Verification items for the finished model (mm, model axes). Face numbers are marked on the shaded views. A direction names the side the tool comes from. Give positions to 0.01 mm unless a question says otherwise; leave off trailing zeros. Loops run counter-clockwise (first coordinate to the right, second up) from the corner with the lowest first, then second, coordinate; pieces in that order, holes last. Notation, with made-up numbers: M 42,51 L 57,51 A17 ccw 57,78 Z; hole C 73.5,16 d3. An arc over 180 degrees is marked long. Use a Markdown table: item, result.
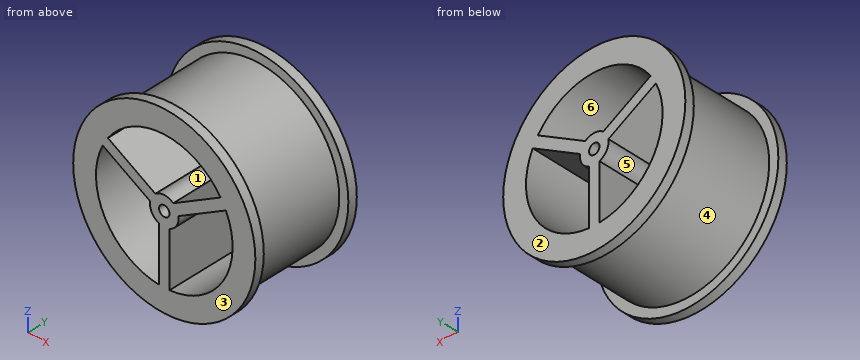
Autodesk Inventor part; units mm, degrees
ref_plane "YZ Plane" through (0, 0, 0) normal (1, 0, 0) x (0, 1, 0)
ref_plane "XZ Plane" through (0, 0, 0) normal (0, 1, 0) x (-1, 0, 0)
ref_plane "XY Plane" through (0, 0, 0) normal (0, 0, 1) x (1, 0, 0)
sketch "Эскиз1" plane through (0, 0, 0) normal (0, 0, 1) x (1, 0, 0)
  line L0 (0, 0) -> (15, 0)
  line L1 (15, 0) -> (15, 10)
  line L2 (15, 10) -> (15, -10)
  line L3 (15, 10) -> (18, 10)
  line L4 (18, 10) -> (18, -10)
  line L5 (18, -10) -> (15, -10)
  line L6 (15, -10) -> (15, 10)
  line L7 (15, 10) -> (20, 10)
  line L8 (20, 10) -> (20, 12)
  line L9 (20, 12) -> (15, 12)
  line L10 (15, 12) -> (15, 10)
  line L11 (15, -10) -> (20, -10)
  line L12 (20, -10) -> (20, -12)
  line L13 (20, -12) -> (15, -12)
  line L14 (15, -12) -> (15, -10)
  line L15 (0, 0) -> (0, 10)
  dimension "d0" = 15
  dimension "d1" = 10
  dimension "d2" = 20
  dimension "d3" = 3
  dimension "d4" = 5
  dimension "d5" = 2
  dimension "d6" = 5
  dimension "d7" = 2
revolve "Вращение1" add sketch "Эскиз1" angle 360 about axis through (0, 0, 0) along (0, 1, 0)
sketch "Эскиз2" plane through (0, -12, 0) normal (0, -1, 0) x (1, 0, 0)
  circle A0 centre (0, 0) radius 1.15
  circle A1 centre (0, 0) radius 3.15
  circle A2 centre (0, 0) radius 15
  line L0 (-1.15, 0) -> (1.15, 0)
  line L1 (1.15, 0) -> (1.15, -15.6419)
  line L2 (1.15, -15.6419) -> (-1.15, -15.6419)
  line L3 (-1.15, -15.6419) -> (-1.15, 0)
  line L4 (14.1213, 6.825) -> (0.575, -0.9959)
  line L5 (-0.575, 0.9959) -> (12.9713, 8.8169)
  line L6 (12.9713, 8.8169) -> (14.1213, 6.825)
  line L7 (0.575, -0.9959) -> (-0.575, 0.9959)
  line L8 (-12.9713, 8.8169) -> (0.575, 0.9959)
  line L9 (-0.575, -0.9959) -> (-14.1213, 6.825)
  line L10 (-14.1213, 6.825) -> (-12.9713, 8.8169)
  line L11 (0.575, 0.9959) -> (-0.575, -0.9959)
  dimension "d9" = 2.3
  dimension "d10" = 2
  dimension "d13" = 360
extrude "Выдавливание1" add sketch "Эскиз2" against normal up to surface (24 mm away) contours L0 L11 A0 | L1 L4 A0 | A0 L7 L0 | A0 L8 L5 A1 L4 L1 | L11 L7 A0 | A0 L5 L8 | L4 L1 A1 L3 L9 A0 | A0 L11 L7 | L11 A0 L0 | L0 A0 L7 | L4 A1 L1 | A0 L3 L9 A1 L8 L5 | L8 A1 L5 | L9 L3 A0 | L1 A2 L3 A1 | A1 L5 A2 L4 | A1 L9 A2 L8 | L3 A1 L9 | L1 L2 L3 A2 | A2 L5 L6 L4 | A2 L9 L10 L8
extrude "Выдавливание2" cut sketch "Эскиз2" against normal up to surface (24 mm away) contours L0 L11 A0 | A0 L7 L0 | L11 L7 A0 | A0 L11 L7 | L11 A0 L0 | L0 A0 L7
properties part number "Wheel down"
(1) Gauge pin test, flat ends, axial feed: P1, Ø12, axis at x = -3.5, y = 9, coming from the -Z side; P2, Ø2, axis at x = -10.5, y = 8, coming from the +Z side; P3, Ø1.5, axis at x = 3, y = -3.5, coming from the -Z side. Record the tip position at first contact, or that the pin passes through.
Results below:
| item | result |
|---|---|
| P1 | z = -20 |
| P2 | z = 15.29 |
| P3 | z = -17.86 |
(2) Cross-section at D-D on z = 9.5. Record the cut outline in (x, y), then the cut area to 3 significant figures.
Results below:
| item | result |
|---|---|
| outline | M -17.6,-12 L -11.61,-12 L -11.61,12 L -17.6,12 L -17.6,10 L -15.29,10 L -15.29,-10 L -17.6,-10 Z; M 11.61,-12 L 17.6,-12 L 17.6,-10 L 15.29,-10 L 15.29,10 L 17.6,10 L 17.6,12 L 11.61,12 Z |
| area | 195 mm^2 |
(3) Cross-section at A-A on x = 0. Record the cut outline in (y, z), then the cut area to 3 significant figures.
Results below:
| item | result |
|---|---|
| outline | M -12,-20 L -10,-20 L -10,-18 L 10,-18 L 10,-20 L 12,-20 L 12,-1.15 L -12,-1.15 Z; M -12,1.15 L 12,1.15 L 12,3.15 L -12,3.15 Z; M -12,15 L 12,15 L 12,20 L 10,20 L 10,18 L -10,18 L -10,20 L -12,20 Z |
| area | 540 mm^2 |
(4) Draft check along Z on the marked faces 3, 4, 5 and 6. Enter one of: +Z half, -Z half, draft (parallel to the pull), parting line (faces both ways), or undercut.
Results below:
| item | result |
|---|---|
| face 3 | draft |
| face 4 | parting line |
| face 5 | undercut |
| face 6 | undercut |
(5) Cross-section at B-B on y = 5.25. Record the cut outline in (x, z), then the cut area to 3 significant figures.
Results below:
| item | result |
|---|---|
| outline | C 0,0 d36; hole M -13.53,6.48 A15 ccw -1.15,-14.96 L -1.15,-2.93 A3.15 cw -3.11,0.47 Z; hole M -12.38,8.47 L -1.96,2.46 A3.15 cw 1.96,2.46 L 12.38,8.47 A15 ccw Z; hole C 0,0 d2.3; hole M 1.15,-14.96 A15 ccw 13.53,6.48 L 3.11,0.47 A3.15 cw 1.15,-2.93 Z |
| area | 420 mm^2 |
(6) Cross-section at C-C on z = -6. Record the cut outline in (x, y), then the cut area to 3 significant figures.
Results below:
| item | result |
|---|---|
| outline | M -19.08,-12 L -13.75,-12 L -13.75,12 L -19.08,12 L -19.08,10 L -16.97,10 L -16.97,-10 L -19.08,-10 Z; M -1.15,-12 L 1.15,-12 L 1.15,12 L -1.15,12 Z; M 13.75,-12 L 19.08,-12 L 19.08,-10 L 16.97,-10 L 16.97,10 L 19.08,10 L 19.08,12 L 13.75,12 Z |
| area | 227 mm^2 |
(7) Set-up check for the marked faces 1 and 2: record each of +Z, -Z, +X, -X, +Y, -Y from which the full face is reachable in a straight line by a thin tool's end or side.
Results below:
| item | result |
|---|---|
| face 1 | +Y, -Y |
| face 2 | +Z, -Z, +X, -X, +Y |
(8) Material ranges on line 1 (Z direction, x = 0, y = 0.5); line 2 (X direction, y = -2.5, z = 0); line 3 (X direction, y = -7.5, z = -2), recorded low to high.
Results below:
| item | result |
|---|---|
| line 1 | -18 to -1.15, 1.15 to 3.15, 15 to 18 |
| line 2 | -18 to -15, -3.15 to -1.15, 1.15 to 3.15, 15 to 18 |
| line 3 | -17.89 to -14.87, -2.43 to 2.43, 14.87 to 17.89 |
